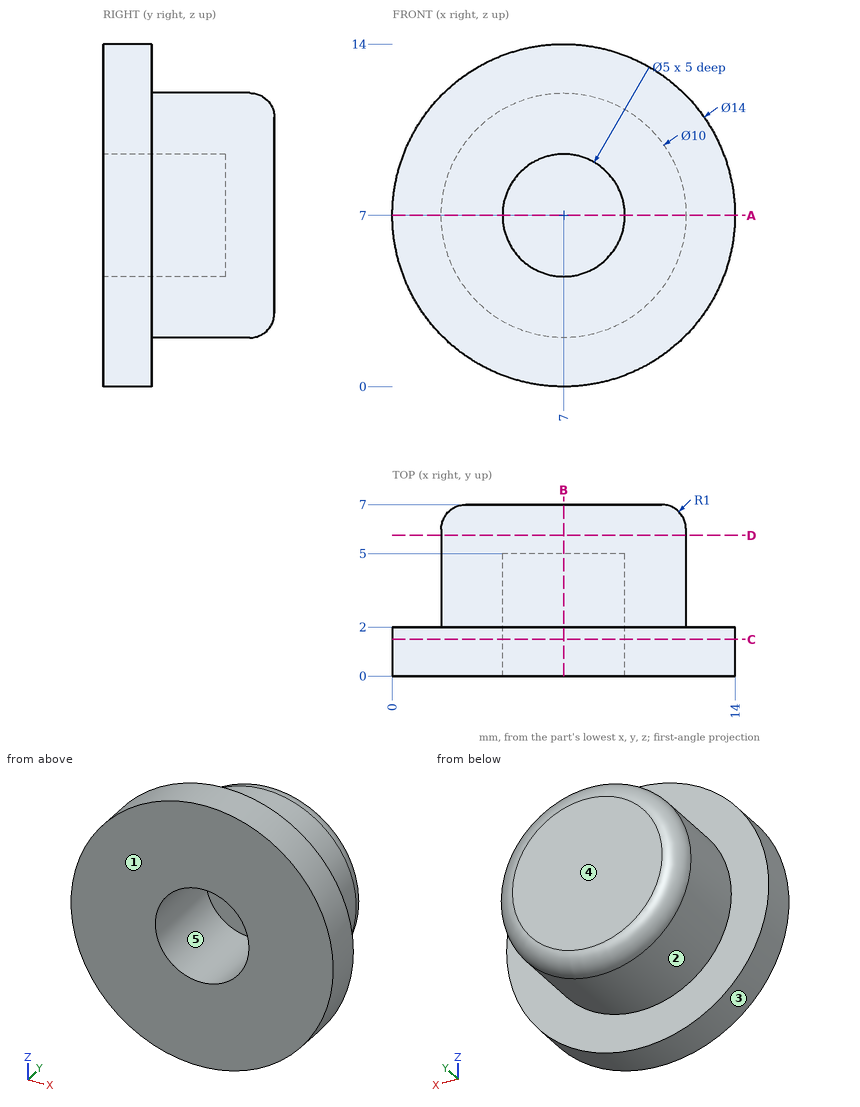
Geometry: see drawing. Coordinates: mm, zero at the bounding-box minimum. A direction names the side the tool comes from. Round coordinates to 2 decimals unless told otherwise and drop trailing zeros. Write each loop counter-clockwise with the first axis right and the second up, starting at its lowest first coordinate (ties: lowest second). Pieces come first, ordered by that corner, then holes. Notation, with made-up numbers: (56, 12.5) - (61, 12.5) arc R28 ccw to (61, 34.5) - close; hole circle Ø8 at (71, -27). An arc over 180 degrees is marked (long way). Use CSV: the item, a comma, the result in double quotes. Start each with the question number.
(1) Cut plane B-B, the plane x = 7. Return loops of the section in (y, z), and give its area (3 significant figures).
(2) Mould query, pull axis X, two halves, no side actions, for the marked faces 3, 4 and 5. Classes: pulls with the +X half, pulls with the -X half, needs draft (parallel to the pull), parting line crosses it, or undercut.
(3) Cut plane C-C, the plane y = 1.5. Return loops of the section in (x, z).
(4) Material intervals for probe 1 along Z at (x, y) = (7, 2.3); probe 2 along Z at (x, y) = (7, 1.3); probe 3 along Y at (x, z) = (8.25, 7.75), sorted ascending. Write a range as [from, to].
(5) Cut plane A-A, the plane z = 7. Return loops of the section in (x, y).
(6) Cut plane D-D, the plane y = 5.75. Return loops of the section in (x, z), and give its area (3 significant figures).
(7) Set-up query: the marked faces 1 and 2. Return all of +Z, -Z, +X, -X, +Y, -Y with unobstructed straight access to the full face (end or side cutting, diameter ignored); none if empty.
(8) First-contact query: pin 1 Ø5 at (x, z) = (10.5, 10) entering from -Y; pin 2 Ø1 at (x, y) = (8, 2) entering from +Z; pin 3 Ø1.5 at (x, y) = (7, 4) entering from +Z; pin 4 Ø1 at (y, z) = (2, 6) entering from -X. Flat tips, straight axial feed; report the tip coordinate or a pass-through.
Geometry says:
1,outline,"(0, 0) - (2, 0) - (2, 2) - (6, 2) arc R1 ccw to (7, 3) - (7, 11) arc R1 ccw to (6, 12) - (2, 12) - (2, 14) - (0, 14) - (0, 9.5) - (5, 9.5) - (5, 4.5) - (0, 4.5) - close"
1,area,"52.6 mm²"
2,face 3,"parting line crosses it"
2,face 4,"needs draft"
2,face 5,"undercut"
3,outline,"circle Ø14 at (7, 7); hole circle Ø5 at (7, 7)"
4,probe 1,"[2, 4.5], [9.5, 12]"
4,probe 2,"[0, 4.5], [9.5, 14]"
4,probe 3,"[5, 7]"
5,outline,"(0, 0) - (4.5, 0) - (4.5, 5) - (9.5, 5) - (9.5, 0) - (14, 0) - (14, 2) - (12, 2) - (12, 6) arc R1 ccw to (11, 7) - (3, 7) arc R1 ccw to (2, 6) - (2, 2) - (0, 2) - close"
6,outline,"circle Ø10 at (7, 7)"
6,area,"78.5 mm²"
7,face 1,"+Z, -Z, +X, -X, -Y"
7,face 2,"+Y"
8,pin 1,"y = 0"
8,pin 2,"z = 13.98"
8,pin 3,"z = 12"
8,pin 4,"x = 0.02"
